Work out the finished part from the listing and answer in its coordinate system (mm). Face numbers are marked on the shaded views. A direction names the side the tool comes from. Coordinates: 2 decimals unless noted, no trailing zeros. Order: outer loops, then holes, each group sorted by start corner. A loop starts at its lowest first (then second) coordinate and runs counter-clockwise, first axis right, second up. Notation, with made-up numbers: M 22,-35 L 62,-35 A12 ccw 62,-13 Z; hole C 88.25,-2 d1. An arc over 180 degrees is marked long. Use a Markdown table: item, result.
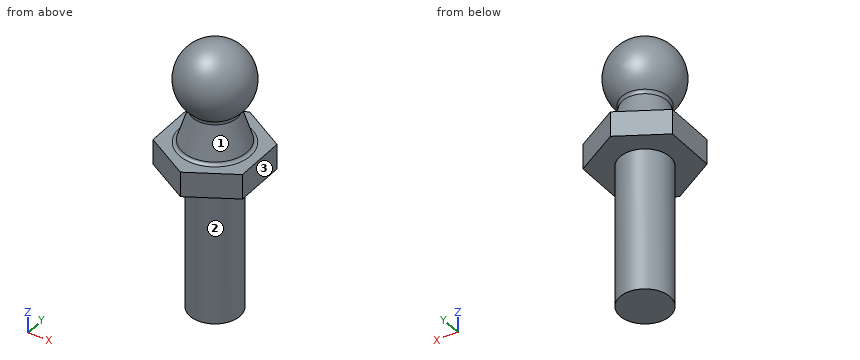
from build123d import *

# Parameters (mm, degrees)
BOSS_EXTRUDE2_DEPTH = 3.5
SKETCH3_R           = 3.5
BOSS_EXTRUDE3_DEPTH = 20
FILLET1_R           = 0.5


with BuildPart() as part:
    # Sketch2 → Boss-Extrude2 (new body)
    with BuildSketch(Plane.XY):
        Polygon((0, 7.216878365), (-6.25, 3.608439182), (-6.25, -3.608439182), (0, -7.216878365), (6.25, -3.608439182), (6.25, 3.608439182), align=None)
    extrude(amount=BOSS_EXTRUDE2_DEPTH)

    # Sketch3 → Boss-Extrude3 (add)
    with BuildSketch(Plane(origin=(0, 0, 0), x_dir=(-1, 0, 0), z_dir=(0, 0, -1))):
        Circle(SKETCH3_R)
    extrude(amount=BOSS_EXTRUDE3_DEPTH)

    # Sketch4 → Revolve1 (revolve)
    with BuildSketch(Plane(origin=(0, 0, 0), x_dir=(0, 0, -1), z_dir=(1, 0, 0))):
        with BuildLine():
            Line((-3.5, 0), (-17.5, 0))
            ThreePointArc((-17.5, 0), (-14.08113883, 4.74341649), (-8.5, 3))
            Line((-8.5, 3), (-3.5, 4.6))
            Line((-3.5, 4.6), (-3.5, 0))
        make_face()
    revolve(axis=Axis((0, 0, 3.5), (0, 0, 1)))

    # Fillet1
    fillet1_edges = [part.edges().sort_by_distance(p)[0] for p in [
        (0, -4.6, 3.5),
        (0, -3, 8.5),
    ]]
    fillet(fillet1_edges, radius=FILLET1_R)


solid = part.part
1. For the marked faces 1, 2 and 3, determine the directions among +Z, -Z, +X, -X, +Y, -Y from which every point of the face is accessible in a straight line to the end or side of a thin tool.
Answers below:
| item | result |
|---|---|
| face 1 | none |
| face 2 | -Z |
| face 3 | +Z, -Z, +X, +Y, -Y |
2. Flat-ended cylindrical pins translate along their axes: P1, Ø3, axis at x = 4, y = 0.5, coming from the +Z side; P2, Ø3, axis at x = 3, z = -11.5, coming from the +Y side; P3, Ø1.5, axis at y = 1, z = -2, coming from the +X side; P4, Ø1.5, axis at y = 5.5, z = -4.5, coming from the -X side. Find the tip coordinate at first contact, or state that the pin passes through.
Answers below:
| item | result |
|---|---|
| P1 | z = 16.81 |
| P2 | y = 3.16 |
| P3 | x = 3.49 |
| P4 | through |
3. Section C-C on z = 4.5 is taken. Determine the outline of the cut face in (x, y).
Answers below:
| item | result |
|---|---|
| outline | C 0,0 d8.56 |
4. Section B-B on y = -5.5 is taken. Determine the outline of the cut face in (x, z), then the cut area to 3 significant figures.
Answers below:
| item | result |
|---|---|
| outline | M -2.97,0 L 2.97,0 L 2.97,3.5 L -2.97,3.5 Z |
| area | 20.8 mm² |
5. Find the intervals of material crossed by probe 1 along Y at (x, z) = (0, -6.5); probe 2 along Z at (x, y) = (-3.75, -4.25); probe 3 along Y at (x, z) = (1, 7.5), in increasing order.
Answers below:
| item | result |
|---|---|
| probe 1 | -3.5 to 3.5 |
| probe 2 | 0 to 3.5 |
| probe 3 | -3.17 to 3.17 |
6. Section A-A on z = -15.5 is taken. Determine the outline of the cut face in (x, y), then the cut area to 3 significant figures.
Answers below:
| item | result |
|---|---|
| outline | C 0,0 d7 |
| area | 38.5 mm² |
